Job drawing, mm, ordinate dimensions from the low corner. One solid piece. A direction names the side the tool comes from. Coordinates: 2 decimals unless noted, no trailing zeros. Loops run counter-clockwise (first coordinate to the right, second up) from the corner with the lowest first, then second, coordinate; pieces in that order, holes last. Notation, with made-up numbers: (73.25, 70.25) - (118.25, 70.25) arc R13 cw to (118.25, 78.25) - close; hole circle Ø1 at (20.5, -16.5). An arc over 180 degrees is marked (long way). Use a Markdown table: item, result. Add a question column.
1) Band-saw the part on A-A (x = 8). Give the cut face in (y, z), plus the area to 3 significant figures.
2) Band-saw the part on D-D (z = 11.25). Give the cut face in (x, y).
3) Drop flat-ended pins along their axis: P1, Ø1.5, axis at x = 3.5, y = 5.5, coming from the -Z side (3 decimals); P2, Ø2, axis at y = 9.5, z = 6.5, coming from the +X side; P3, Ø4, axis at x = 4, y = 14, coming from the -Z side. Give the stop position or say it passes through.
4) Probe probe 1 along X at (y, z) = (4.75, 8); probe 2 along Y at (x, z) = (13.25, 4.25); probe 3 along Y at (x, z) = (13, 13.5). List the from-to ranges inside material, lowest first. Write a range as [from, to].
5) Band-saw the part on C-C (y = 13). Give the cut face in (x, z), plus the area to 3 significant figures.
6) Band-saw the part on B-B (z = 8). Give the cut face in (x, y).
7) Tool access for the marked faces 1, 2 and 3: list every direction of +Z, -Z, +X, -X, +Y, -Y with a clear straight run to the whole face (end or side of a thin tool).
8) Pull direction Z, two halves, no side cores. Call the marked faces 4, 5 and 6: +Z half, -Z half, draft (parallel to the pull), parting line (faces both ways), or undercut.
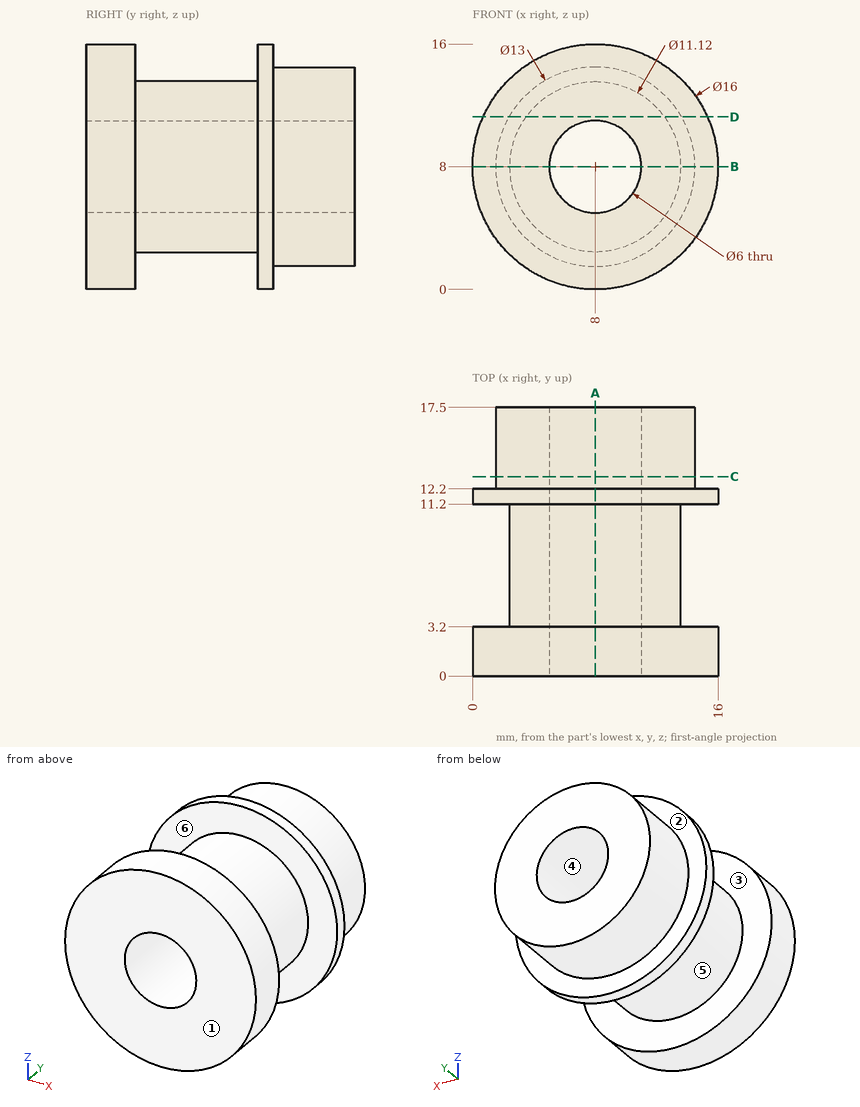
Answer block:
| question | item | result |
|---|---|---|
| 1 | outline | (0, 0) - (3.2, 0) - (3.2, 2.44) - (11.2, 2.44) - (11.2, 0) - (12.2, 0) - (12.2, 1.5) - (17.5, 1.5) - (17.5, 5) - (0, 5) - close; (0, 11) - (17.5, 11) - (17.5, 14.5) - (12.2, 14.5) - (12.2, 16) - (11.2, 16) - (11.2, 13.56) - (3.2, 13.56) - (3.2, 16) - (0, 16) - close |
| 1 | area | 120 mm2 |
| 2 | outline | (0.69, 0) - (15.31, 0) - (15.31, 3.2) - (12.51, 3.2) - (12.51, 11.2) - (15.31, 11.2) - (15.31, 12.2) - (13.63, 12.2) - (13.63, 17.5) - (2.37, 17.5) - (2.37, 12.2) - (0.69, 12.2) - (0.69, 11.2) - (3.49, 11.2) - (3.49, 3.2) - (0.69, 3.2) - close |
| 3 | P1 | z = 3.895 |
| 3 | P2 | x = 13.54 |
| 3 | P3 | z = 0.64 |
| 4 | probe 1 | [2.44, 5], [11, 13.56] |
| 4 | probe 2 | [0, 3.2], [11.2, 17.5] |
| 4 | probe 3 | [0, 3.2], [11.2, 12.2] |
| 5 | outline | circle Ø13 at (8, 8); hole circle Ø6 at (8, 8) |
| 5 | area | 104 mm2 |
| 6 | outline | (0, 0) - (5, 0) - (5, 17.5) - (1.5, 17.5) - (1.5, 12.2) - (0, 12.2) - (0, 11.2) - (2.44, 11.2) - (2.44, 3.2) - (0, 3.2) - close; (11, 0) - (16, 0) - (16, 3.2) - (13.56, 3.2) - (13.56, 11.2) - (16, 11.2) - (16, 12.2) - (14.5, 12.2) - (14.5, 17.5) - (11, 17.5) - close |
| 7 | face 1 | +Z, -Z, +X, -X, -Y |
| 7 | face 2 | +Y |
| 7 | face 3 | none |
| 8 | face 4 | undercut |
| 8 | face 5 | parting line |
| 8 | face 6 | draft |
